For this review, take the finished solid that the model builds, in its own axes (mm). Coordinates: 2 decimals unless noted, no trailing zeros. Write each loop counter-clockwise with the first axis right and the second up, starting at its lowest first coordinate (ties: lowest second). Pieces come first, ordered by that corner, then holes. Notation, with made-up numbers: M 62,-40 L 90,-40 A17 cw 90,-36 Z; hole C 80,61 d1. An arc over 180 degrees is marked long. One line per question, with ' | ' between items.
from build123d import *

# Parameters (mm, degrees)
EXTRUDE_1_DEPTH     = 3
SKETCH_3_R          = 4.15
CUT_EXTRUDE_2_DEPTH = 3


with BuildPart() as part:
    # 草图1 → 凸台-拉伸1 (new body)
    with BuildSketch(Plane(origin=(0, 0, 0), x_dir=(1, 0, 0), z_dir=(0, 1, 0))):
        Polygon((14, 20), (-14, 20), (-14, 7.5), (-17, 7.5), (-17, -7.5), (-14, -7.5), (-14, -20), (14, -20), (14, -7.5), (17, -7.5), (17, 7.5), (14, 7.5), align=None)
        with BuildLine():
            ThreePointArc((-5.15, -13), (-5.857106781, -11.292893219), (-4.15, -12))
            Line((-4.15, -12), (4.15, -12))
            ThreePointArc((4.15, -12), (5.857106781, -11.292893219), (5.15, -13))
            Line((5.15, -13), (5.15, -14.3))
            ThreePointArc((5.15, -14.3), (5.857106781, -16.007106781), (4.15, -15.3))
            Line((4.15, -15.3), (-4.15, -15.3))
            ThreePointArc((-4.15, -15.3), (-5.857106781, -16.007106781), (-5.15, -14.3))
            Line((-5.15, -14.3), (-5.15, -13))
        make_face(mode=Mode.SUBTRACT)
        with BuildLine():
            ThreePointArc((-5.15, 14.3), (-5.857106781, 16.007106781), (-4.15, 15.3))
            Line((-4.15, 15.3), (4.15, 15.3))
            ThreePointArc((4.15, 15.3), (5.857106781, 16.007106781), (5.15, 14.3))
            Line((5.15, 14.3), (5.15, 13))
            ThreePointArc((5.15, 13), (5.857106781, 11.292893219), (4.15, 12))
            Line((4.15, 12), (-4.15, 12))
            ThreePointArc((-4.15, 12), (-5.857106781, 11.292893219), (-5.15, 13))
            Line((-5.15, 13), (-5.15, 14.3))
        make_face(mode=Mode.SUBTRACT)
    extrude(amount=EXTRUDE_1_DEPTH)

    # 草图3 → 切除-拉伸2 (cut)
    with BuildSketch(Plane(origin=(0, 3, 0), x_dir=(1, 0, 0), z_dir=(0, 1, 0))):
        with Locations(Location((0, 0, 0), (0, 0, 270))):
            Circle(SKETCH_3_R)
    extrude(amount=-CUT_EXTRUDE_2_DEPTH, mode=Mode.SUBTRACT)


solid = part.part
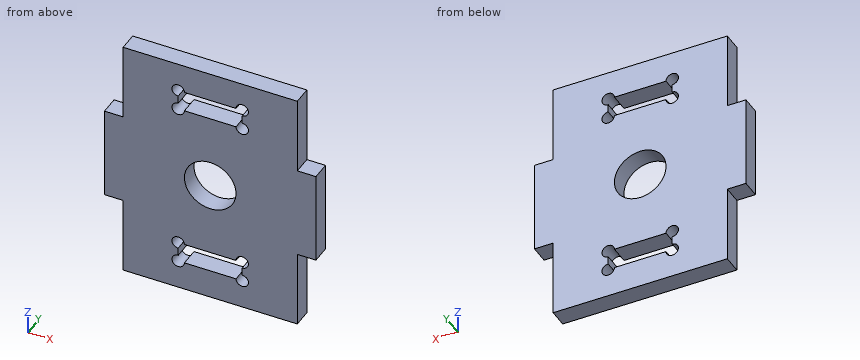
1) To check wall thickness, follow line 1 along Z through (x, y) = (-5, 0.9); line 2 along Z through (x, y) = (3, 2.4); line 3 along Z through (x, y) = (0.5, 0.85). State the ranges of each line that lie inside material, in increasing order. Write a range as [from, to].
Responses:
line 1: [-20, -16.29], [-11.01, 11.01], [16.29, 20] | line 2: [-20, -15.3], [-12, -2.87], [2.87, 12], [15.3, 20] | line 3: [-20, -15.3], [-12, -4.12], [4.12, 12], [15.3, 20]
2) We need section B-B on y = 0.8. State how many separate pieces and enclosed holes the cut face has, then the cut area to 3 significant figures.
Responses:
separate pieces: 1 | enclosed holes: 3 | area: 1,070 mm^2
3) We need section C-C on x = 0. State the section outline as (y, z) points.
Responses:
outline: M 0,-20 L 3,-20 L 3,-15.3 L 0,-15.3 Z; M 0,-12 L 3,-12 L 3,-4.15 L 0,-4.15 Z; M 0,4.15 L 3,4.15 L 3,12 L 0,12 Z; M 0,15.3 L 3,15.3 L 3,20 L 0,20 Z
4) Insertion check: pin 1 Ø1.2 at (x, z) = (-5.15, -15.3) entering from -Y; pin 2 Ø0.9 at (x, y) = (16, 1) entering from -Z; pin 3 Ø1.5 at (y, z) = (1, 12) entering from -X; pin 4 Ø0.7 at (y, z) = (1, -13.5) entering from +X. Each pin has a flat end and moves straight along its axis. Give the tip position at first contact, or say it passes through.
Responses:
pin 1: through | pin 2: z = -7.5 | pin 3: x = -14 | pin 4: x = 14
5) We need section D-D on z = -1. State the section outline as (x, y) points.
Responses:
outline: M -17,0 L -4.03,0 L -4.03,3 L -17,3 Z; M 4.03,0 L 17,0 L 17,3 L 4.03,3 Z
6) We need section A-A on z = -13.5. State the section outline as (x, y) points.
Responses:
outline: M -14,0 L -5.15,0 L -5.15,3 L -14,3 Z; M 5.15,0 L 14,0 L 14,3 L 5.15,3 Z
